Can you work these out from the model? Positions are in its coordinate system, mm. Face numbers are marked on the shaded views. A direction names the side the tool comes from. Give positions to 0.01 mm unless a question says otherwise; leave off trailing zeros. Write each loop counter-clockwise with the first axis right and the second up, starting at its lowest first coordinate (ties: lowest second). Pieces come first, ordered by that corner, then holes.
from build123d import *

# Parameters (mm, degrees)
BRACKET_DEPTH       = 11.5
BOSS_EXTRUDE1_START = -3
BOSS_EXTRUDE1_DEPTH = 3


with BuildPart() as part:
    # Sketch9 → Bracket (new body)
    with BuildSketch(Plane(origin=(0, 0, 0), x_dir=(1, 0, 0), z_dir=(0, 1, 0))):
        with BuildLine():
            Line((5.15, -5), (4.65, -5))
            Line((4.65, -5), (3.35, -5))
            Line((3.35, -5), (3.35, -7))
            Line((3.35, -7), (6.4, -7))
            ThreePointArc((6.4, -7), (6.930330086, -6.780330086), (7.15, -6.25))
            Line((7.15, -6.25), (7.15, -5))
            Line((7.15, -5), (7.15, -3.25))
            ThreePointArc((7.15, -3.25), (7.369669914, -2.719669914), (7.9, -2.5))
            Line((7.9, -2.5), (21.4, -2.5))
            ThreePointArc((21.4, -2.5), (21.930330086, -2.280330086), (22.15, -1.75))
            Line((22.15, -1.75), (22.15, 24.75))
            ThreePointArc((22.15, 24.75), (21.930330086, 25.280330086), (21.4, 25.5))
            Line((21.4, 25.5), (7.9, 25.5))
            ThreePointArc((7.9, 25.5), (7.369669914, 25.719669914), (7.15, 26.25))
            Line((7.15, 26.25), (7.15, 28))
            Line((7.15, 28), (7.15, 29.75))
            ThreePointArc((7.15, 29.75), (6.930330086, 30.280330086), (6.4, 30.5))
            Line((6.4, 30.5), (5.15, 30.5))
            Line((5.15, 30.5), (3.35, 30.5))
            Line((3.35, 30.5), (3.35, 28.5))
            Line((3.35, 28.5), (5.15, 28.5))
            Line((5.15, 28.5), (5.15, 28))
            Line((5.15, 28), (5.15, 23.5))
            Line((5.15, 23.5), (20.15, 23.5))
            Line((20.15, 23.5), (20.15, -0.5))
            Line((20.15, -0.5), (5.15, -0.5))
            Line((5.15, -0.5), (5.15, -5))
        make_face()
    extrude(amount=BRACKET_DEPTH)

    # Sketch12 → Boss-Extrude1 (add)
    with BuildSketch(Plane(origin=(0, 0, 0), x_dir=(1, 0, 0), z_dir=(0, 1, 0)).offset(BOSS_EXTRUDE1_START)):
        with BuildLine():
            Line((3.134136634, -6.799408153), (-15.169112008, 10.208954707))
            ThreePointArc((-15.169112008, 10.208954707), (-17.445237733, 24.907700028), (-3.6745965, 30.529381479))
            ThreePointArc((-3.6745965, 30.529381479), (-3.571695801, 30.507381696), (-3.466728879, 30.5))
            Line((-3.466728879, 30.5), (6.4, 30.5))
            ThreePointArc((6.4, 30.5), (6.930330086, 30.280330086), (7.15, 29.75))
            Line((7.15, 29.75), (7.15, 26.25))
            ThreePointArc((7.15, 26.25), (7.369669914, 25.719669914), (7.9, 25.5))
            Line((7.9, 25.5), (21.4, 25.5))
            ThreePointArc((21.4, 25.5), (21.930330086, 25.280330086), (22.15, 24.75))
            Line((22.15, 24.75), (22.15, -1.75))
            ThreePointArc((22.15, -1.75), (21.930330086, -2.280330086), (21.4, -2.5))
            Line((21.4, -2.5), (7.9, -2.5))
            ThreePointArc((7.9, -2.5), (7.369669914, -2.719669914), (7.15, -3.25))
            Line((7.15, -3.25), (7.15, -6.25))
            ThreePointArc((7.15, -6.25), (6.930330086, -6.780330086), (6.4, -7))
            Line((6.4, -7), (3.644676233, -7))
            ThreePointArc((3.644676233, -7), (3.370410043, -6.948053048), (3.134136634, -6.799408153))
        make_face()
    extrude(amount=BOSS_EXTRUDE1_DEPTH)


solid = part.part
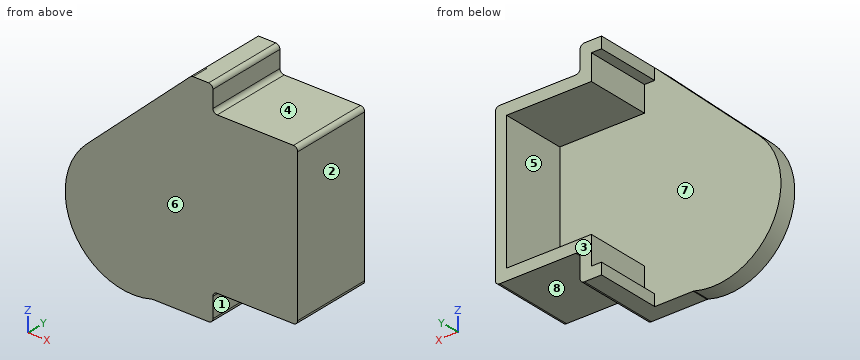
(1) Imagine slicing it at B-B, the plane x = 18.5. Write out the boundary of the cut face in (y, z), plus the area to 3 significant figures.
Returned:
outline: (-3, -25.5) - (11.5, -25.5) - (11.5, -23.5) - (0, -23.5) - (0, 0.5) - (11.5, 0.5) - (11.5, 2.5) - (-3, 2.5) - close
area: 130 mm2
(2) Will these pins go through, and if not, where does the flat tip stop? P1, Ø19, axis at x = -8, z = -4, coming from the +Y side; P2, Ø1.4, axis at x = 4.5, y = 4.5, coming from the -Z side; P3, Ø6.5, axis at x = 14, y = 4, coming from the -Z side.
Returned:
P1: stops at y = 0
P2: stops at z = -30.5
P3: stops at z = -25.5
(3) If we mould it in two halves opening along Z, with no side actions, what happens to the marked faces 6, 7 and 8? For each: +Z half, -Z half, draft (parallel to the pull), parting line (faces both ways), or undercut.
Returned:
face 6: draft
face 7: undercut
face 8: -Z half
(4) For the marked faces 1, 2, 3, 4 and 5, which set-ups out of +Z, -Z, +X, -X, +Y, -Y let a thin tool reach every point of the face, with its end or its side?
Returned:
face 1: -Z, +X, +Y, -Y
face 2: +Z, -Z, +X, +Y, -Y
face 3: +Z, -Z, +X, -X, +Y
face 4: +Z, +X, +Y, -Y
face 5: -X, +Y
(5) If I drill on L1, parallel to Z at x = 5.5, y = 2.25; L2, parallel to Z at x = 14.5, y = 3.5; L3, parallel to X at y = 9.25, z = 0, over which ranges is the centre line in solid material (lowest first)?
Returned:
L1: z = -30.5 to -23.5, 0.5 to 7
L2: z = -25.5 to -23.5, 0.5 to 2.5
L3: x = 20.15 to 22.15
(6) Imagine slicing it at D-D, the plane z = 4. Write out the boundary of the cut face in (x, y), plus the area to 3 significant figures.
Returned:
outline: (0.12, -3) - (7.15, -3) - (7.15, 11.5) - (5.15, 11.5) - (5.15, 0) - (0.12, 0) - close
area: 44.1 mm2
(7) Imagine slicing it at C-C, the plane z = -19. Write out the boundary of the cut face in (x, y), plus the area to 3 significant figures.
Returned:
outline: (-19, -3) - (22.15, -3) - (22.15, 11.5) - (20.15, 11.5) - (20.15, 0) - (-19, 0) - close
area: 146 mm2
(8) Imagine slicing it at A-A, the plane y = 6. Write out the boundary of the cut face in (x, z), plus the area to 3 significant figures.
Returned:
outline: (3.35, -30.5) - (6.4, -30.5) arc R0.75 ccw to (7.15, -29.75) - (7.15, -26.25) arc R0.75 cw to (7.9, -25.5) - (21.4, -25.5) arc R0.75 ccw to (22.15, -24.75) - (22.15, 1.75) arc R0.75 ccw to (21.4, 2.5) - (7.9, 2.5) arc R0.75 cw to (7.15, 3.25) - (7.15, 6.25) arc R0.75 ccw to (6.4, 7) - (3.35, 7) - (3.35, 5) - (5.15, 5) - (5.15, 0.5) - (20.15, 0.5) - (20.15, -23.5) - (5.15, -23.5) - (5.15, -28.5) - (3.35, -28.5) - close
area: 142 mm2
